Work out the finished part from the listing and answer in its coordinate system (mm). A direction names the side the tool comes from. Round coordinates to 2 decimals unless told otherwise and drop trailing zeros. Order: outer loops, then holes, each group sorted by start corner. A loop starts at its lowest first (then second) coordinate and runs counter-clockwise, first axis right, second up. Notation, with made-up numbers: (30.5, -23.75) - (80.5, -23.75) arc R28 ccw to (80.5, -4.75) - close; hole circle Ø1 at (-8, 47.5). An arc over 180 degrees is marked (long way). Use CSV: the item, a comma, the result in double quotes.
from build123d import *

# Parameters (mm, degrees)
F0_W     = 101.6
F0_H     = 18.288
F1_DEPTH = 12.7
F2_W     = 101.6
F2_H     = 18.288
F4_DEPTH = 25.4
F3_W     = 101.6
F3_H     = 18.288
F5_DEPTH = 25.4
F6_R     = 1.27
F7_R     = 5.08


with BuildPart() as f1:
    # F0 (on Top) → F1 (new body, symmetric)
    with BuildSketch(Plane.XY):
        Rectangle(F0_W, F0_H)
    extrude(amount=F1_DEPTH, both=True)

    # F2 (on face) → F4 (join)
    with BuildSketch(Plane(origin=(0, 0, -12.7), x_dir=(1, 0, 0), z_dir=(0, 0, -1))):
        Rectangle(F2_W, F2_H)
        with BuildLine():
            Line((-42.3926, 2.956892), (-42.3926, 6.35))
            Line((-42.3926, 6.35), (42.3926, 6.35))
            Line((42.3926, 6.35), (42.3926, 2.956892))
            ThreePointArc((42.3926, 2.956892), (44.6278, 0), (42.3926, -2.956892))
            Line((42.3926, -2.956892), (42.3926, -6.35))
            Line((42.3926, -6.35), (-42.3926, -6.35))
            Line((-42.3926, -6.35), (-42.3926, -2.956892))
            ThreePointArc((-42.3926, -2.956892), (-44.6278, 0), (-42.3926, 2.956892))
        make_face(mode=Mode.SUBTRACT)
    extrude(amount=F4_DEPTH)

    # F3 (on face) → F5 (join)
    with BuildSketch(Plane.XY.offset(12.7)):
        Rectangle(F3_W, F3_H)
        with BuildLine():
            Line((-42.3926, 2.956892), (-42.3926, 6.35))
            Line((-42.3926, 6.35), (42.3926, 6.35))
            Line((42.3926, 6.35), (42.3926, 2.956892))
            ThreePointArc((42.3926, 2.956892), (44.6278, 0), (42.3926, -2.956892))
            Line((42.3926, -2.956892), (42.3926, -6.35))
            Line((42.3926, -6.35), (-42.3926, -6.35))
            Line((-42.3926, -6.35), (-42.3926, -2.956892))
            ThreePointArc((-42.3926, -2.956892), (-44.6278, 0), (-42.3926, 2.956892))
        make_face(mode=Mode.SUBTRACT)
    extrude(amount=F5_DEPTH)

    # F6
    f6_edges = [f1.edges().sort_by_distance(p)[0] for p in [
        (-42.3926, -2.956892, -25.4),
        (-42.3926, 2.956892, -25.4),
        (42.3926, -2.956892, -25.4),
        (42.3926, 2.956892, -25.4),
        (42.3926, -2.956892, 25.4),
        (42.3926, 2.956892, 25.4),
        (-42.3926, -2.956892, 25.4),
        (-42.3926, 2.956892, 25.4),
    ]]
    fillet(f6_edges, radius=F6_R)

    # F7
    f7_edges = [f1.edges().sort_by_distance(p)[0] for p in [
        (50.8, -9.144, 0),
        (50.8, 9.144, 0),
        (-50.8, -9.144, 0),
        (-50.8, 9.144, 0),
    ]]
    fillet(f7_edges, radius=F7_R)


solid = f1.part
(1) Find the intervals of material crossed by L1, parallel to X at y = 3.75, z = -34; L2, parallel to Y at x = 5, z = -33.5; L3, parallel to Z at x = -28, y = 3.75, in increasing order. Write a range as from..to.
Findings below:
L1,"x = -50.8..-42.39, 42.39..50.8"
L2,"y = -9.14..-6.35, 6.35..9.14"
L3,"z = -12.7..12.7"
(2) For faces 1 (the flat face through (42.393, 5, 25)), 2 (the cylindrical face through (49.27, -7.7, 0.53)), 3 (the cylindrical face through (-44.627, 0.046, -25.222)), determine the directions among +Z, -Z, +X, -X, +Y, -Y from which every point of the face is accessible in a straight line to the end or side of a thin tool.
Findings below:
face 1,"+Z"
face 2,"+Z, -Z, +X, -Y"
face 3,"-Z"
(3) Find section B-B (x = -10). Determine the outline of the cut face in (y, z), and give its area (3 significant figures).
Findings below:
outline,"(-9.14, -38.1) - (-6.35, -38.1) - (-6.35, -12.7) - (6.35, -12.7) - (6.35, -38.1) - (9.14, -38.1) - (9.14, 38.1) - (6.35, 38.1) - (6.35, 12.7) - (-6.35, 12.7) - (-6.35, 38.1) - (-9.14, 38.1) - close"
area,"748 mm²"
(4) Each of these flat-tipped pins is pushed along its axis until it touches: pin 1 (0.8 mm diameter, centred on y = 5.5, z = -20, fed in from -X); pin 2 (0.8 mm diameter, centred on y = 5, z = 19, fed in from -X); pin 3 (0.8 mm diameter, centred on y = -5, z = 30.5, fed in from +X). Where does it stop, or does it pass through?
Findings below:
pin 1,"stops at x = -50.69"
pin 2,"stops at x = -50.77"
pin 3,"stops at x = 50.77"
(5) Find section C-C (y = -1). Determine the outline of the cut face in (x, z), and give its area (3 significant figures).
Findings below:
outline,"(-50.8, -38.1) - (-44.46, -38.1) - (-44.46, -12.7) - (44.46, -12.7) - (44.46, -38.1) - (50.8, -38.1) - (50.8, 38.1) - (44.46, 38.1) - (44.46, 12.7) - (-44.46, 12.7) - (-44.46, 38.1) - (-50.8, 38.1) - close"
area,"3,220 mm²"
(6) Find section A-A (z = -19.5). Determine the outline of the cut face in (x, y).
Findings below:
outline,"(-50.8, -4.06) arc R5.08 ccw to (-45.72, -9.14) - (45.72, -9.14) arc R5.08 ccw to (50.8, -4.06) - (50.8, 4.06) arc R5.08 ccw to (45.72, 9.14) - (-45.72, 9.14) arc R5.08 ccw to (-50.8, 4.06) - close; hole (-43.05, -2.69) arc R1.27 cw to (-42.39, -3.8) - (-42.39, -6.35) - (42.39, -6.35) - (42.39, -3.8) arc R1.27 cw to (43.05, -2.69) arc R3.07 ccw to (43.05, 2.69) arc R1.27 cw to (42.39, 3.8) - (42.39, 6.35) - (-42.39, 6.35) - (-42.39, 3.8) arc R1.27 cw to (-43.05, 2.69) arc R3.07 ccw to start"
(7) The mould has two halves that part along Y. Classify faces 4 (the cylindrical face through (49.27, 7.7, -0.53)), 5 (the flat face through (-1, 6.35, 25)), 6 (the cylindrical face through (-49.35, -7.62, 0.53)): released by +Y, released by -Y, zero draft, split by the parting line, or undercut.
Findings below:
face 4,"released by +Y"
face 5,"undercut"
face 6,"released by -Y"
